For this review, take the finished solid that the model builds, in its own axes (mm). Face numbers are marked on the shaded views. A direction names the side the tool comes from. Give positions to 0.01 mm unless a question says otherwise; leave off trailing zeros. Loops run counter-clockwise (first coordinate to the right, second up) from the corner with the lowest first, then second, coordinate; pieces in that order, holes last. Notation, with made-up numbers: (-7.75, 27.25) - (3.25, 27.25) arc R21 ccw to (3.25, 58.25) - close; hole circle Ø3 at (72.25, 51.25). An arc over 180 degrees is marked (long way). Put each result on its own line as item: value.
from build123d import *

# Parameters (mm, degrees)
EXTRUDE_1_DEPTH     = 1.5
EXTRUDE_3_DEPTH     = 14
SKETCH_4_R          = 1.1
EXTRUDE_4_DEPTH     = 3.2
SKETCH_5_R          = 1.1
EXTRUDE_5_DEPTH     = 3.2
SKETCH_8_R          = 1.1
EXTRUDE_7_DEPTH     = 3.2
SKETCH_9_R          = 0.6
CUT_EXTRUDE_5_DEPTH = 1.5
CUT_EXTRUDE_6_DEPTH = 1.5
CUT_EXTRUDE_7_REACH = 88.953
SKETCH_16_R         = 3.5
FILLET_1_R          = 1


with BuildPart() as part:
    # 草图1 → 凸台-拉伸1 (new body)
    with BuildSketch(Plane.XY):
        with BuildLine():
            Line((-3.146845785, 60.5), (38.953154215, 60.5))
            ThreePointArc((38.953154215, 60.5), (45.458536602, 57.805382387), (48.153154215, 51.3))
            Line((48.153154215, 51.3), (48.153154215, 9.2))
            ThreePointArc((48.153154215, 9.2), (45.458536602, 2.694617613), (38.953154215, 0))
            Line((38.953154215, 0), (-3.146845785, 0))
            ThreePointArc((-3.146845785, 0), (-9.652228172, 2.694617613), (-12.346845785, 9.2))
            Line((-12.346845785, 9.2), (-12.346845785, 51.3))
            ThreePointArc((-12.346845785, 51.3), (-9.652228172, 57.805382387), (-3.146845785, 60.5))
        make_face()
    extrude(amount=EXTRUDE_1_DEPTH)

    # 草图3 → 凸台-拉伸3 (add)
    with BuildSketch(Plane.XY.offset(1.5)):
        with BuildLine():
            Line((38.953154215, 60.5), (-3.146845785, 60.5))
            ThreePointArc((-3.146845785, 60.5), (-9.652228172, 57.805382387), (-12.346845785, 51.3))
            Line((-12.346845785, 51.3), (-12.346845785, 9.2))
            ThreePointArc((-12.346845785, 9.2), (-9.652228172, 2.694617613), (-3.146845785, 0))
            Line((-3.146845785, 0), (38.953154215, 0))
            ThreePointArc((38.953154215, 0), (45.458536602, 2.694617613), (48.153154215, 9.2))
            Line((48.153154215, 9.2), (48.153154215, 51.3))
            ThreePointArc((48.153154215, 51.3), (45.458536602, 57.805382387), (38.953154215, 60.5))
        make_face()
        with BuildLine():
            Line((38.953154215, 59), (-3.146845785, 59))
            ThreePointArc((-3.146845785, 59), (-8.591568001, 56.744722215), (-10.846845785, 51.3))
            Line((-10.846845785, 51.3), (-10.846845785, 9.2))
            ThreePointArc((-10.846845785, 9.2), (-8.591568001, 3.755277785), (-3.146845785, 1.5))
            Line((-3.146845785, 1.5), (38.953154215, 1.5))
            ThreePointArc((38.953154215, 1.5), (44.39787643, 3.755277785), (46.653154215, 9.2))
            Line((46.653154215, 9.2), (46.653154215, 51.3))
            ThreePointArc((46.653154215, 51.3), (44.39787643, 56.744722215), (38.953154215, 59))
        make_face(mode=Mode.SUBTRACT)
    extrude(amount=EXTRUDE_3_DEPTH)

    # 草图4 → 凸台-拉伸4 (add)
    with BuildSketch(Plane.XY.offset(1.5)):
        with BuildLine():
            Line((0, 52), (0, 59))
            Line((0, 59), (-3.146845785, 59))
            ThreePointArc((-3.146845785, 59), (-8.591568001, 56.744722215), (-10.846845785, 51.3))
            Line((-10.846845785, 51.3), (-10.846845785, 49))
            Line((-10.846845785, 49), (-3, 49))
            ThreePointArc((-3, 49), (-0.878679656, 49.878679656), (0, 52))
        make_face()
        with Locations((-4.646845785, 52.8)):
            Circle(SKETCH_4_R, mode=Mode.SUBTRACT)
    extrude(amount=EXTRUDE_4_DEPTH)

    # 草图5 → 凸台-拉伸5 (add)
    with BuildSketch(Plane.XY.offset(1.5)):
        with BuildLine():
            Line((-4.846845785, 10.5), (-10.846845785, 10.5))
            Line((-10.846845785, 10.5), (-10.846845785, 9.2))
            ThreePointArc((-10.846845785, 9.2), (-8.591568001, 3.755277785), (-3.146845785, 1.5))
            Line((-3.146845785, 1.5), (-1.846845785, 1.5))
            Line((-1.846845785, 1.5), (-1.846845785, 7.5))
            ThreePointArc((-1.846845785, 7.5), (-2.725525442, 9.621320344), (-4.846845785, 10.5))
        make_face()
        with Locations((-4.646845785, 8.3)):
            Circle(SKETCH_5_R, mode=Mode.SUBTRACT)
    extrude(amount=EXTRUDE_5_DEPTH)

    # 草图8 → 凸台-拉伸7 (add)
    with BuildSketch(Plane.XY.offset(1.5)):
        with BuildLine():
            Line((37.653154215, 7.5), (37.653154215, 1.5))
            Line((37.653154215, 1.5), (38.953154215, 1.5))
            ThreePointArc((38.953154215, 1.5), (44.39787643, 3.755277785), (46.653154215, 9.2))
            Line((46.653154215, 9.2), (46.653154215, 10.5))
            Line((46.653154215, 10.5), (40.653154215, 10.5))
            ThreePointArc((40.653154215, 10.5), (38.531833871, 9.621320344), (37.653154215, 7.5))
        make_face()
        with Locations((40.453154215, 8.3)):
            Circle(SKETCH_8_R, mode=Mode.SUBTRACT)
    extrude(amount=EXTRUDE_7_DEPTH)

    # 草图9 → 切除-拉伸5 (cut)
    with BuildSketch(Plane.ZY.offset(12.346845785)):
        with Locations(Location((8, 32.8, 0), (0, 0, 270))):
            Circle(SKETCH_9_R)
    extrude(amount=-CUT_EXTRUDE_5_DEPTH, mode=Mode.SUBTRACT)

    # 草图10 → 切除-拉伸6 (cut)
    with BuildSketch(Plane.ZY.offset(12.346845785)):
        with BuildLine():
            Line((9.5, 20.4), (9.5, 14.4))
            ThreePointArc((9.5, 14.4), (7.75, 12.65), (6, 14.4))
            Line((6, 14.4), (6, 20.4))
            ThreePointArc((6, 20.4), (7.75, 22.15), (9.5, 20.4))
        make_face()
    extrude(amount=-CUT_EXTRUDE_6_DEPTH, mode=Mode.SUBTRACT)

    # 草图16 → 切除-拉伸7 (cut, up to next)
    with BuildSketch(Plane(origin=(48.153154215, 0, 0), x_dir=(0, 0, -1), z_dir=(1, 0, 0)), mode=Mode.PRIVATE) as cut_extrude_7_sk1:
        with Locations((-9.65, 27.1)):
            Circle(SKETCH_16_R)
    cut_extrude_7_tool1 = extrude(cut_extrude_7_sk1.sketch, amount=-CUT_EXTRUDE_7_REACH, mode=Mode.PRIVATE) & part.part
    # 草图16 → 切除-拉伸7 (cut, up to next)
    with BuildSketch(Plane(origin=(48.153154215, 0, 0), x_dir=(0, 0, -1), z_dir=(1, 0, 0)), mode=Mode.PRIVATE) as cut_extrude_7_sk2:
        with BuildLine():
            Line((-12, 40.8), (-8, 40.8))
            ThreePointArc((-8, 40.8), (-6.585786438, 40.214213562), (-6, 38.8))
            Line((-6, 38.8), (-6, 35))
            ThreePointArc((-6, 35), (-6.585786438, 33.585786438), (-8, 33))
            Line((-8, 33), (-12, 33))
            ThreePointArc((-12, 33), (-13.414213562, 33.585786438), (-14, 35))
            Line((-14, 35), (-14, 38.8))
            ThreePointArc((-14, 38.8), (-13.414213562, 40.214213562), (-12, 40.8))
        make_face()
    cut_extrude_7_tool2 = extrude(cut_extrude_7_sk2.sketch, amount=-CUT_EXTRUDE_7_REACH, mode=Mode.PRIVATE) & part.part
    add(cut_extrude_7_tool1.solids().sort_by_distance((48.153154, 27.1, 9.65))[0], mode=Mode.SUBTRACT)
    add(cut_extrude_7_tool2.solids().sort_by_distance((48.153154, 36.9, 10))[0], mode=Mode.SUBTRACT)

    # 圆角1
    fillet_1_edges = [part.edges().sort_by_distance(p)[0] for p in [
        (-12.346845785, 30.25, 0),
        (-9.652228172, 57.805382387, 0),
        (17.903154215, 60.5, 0),
        (45.458536602, 57.805382387, 0),
        (48.153154215, 30.25, 0),
        (45.458536602, 2.694617613, 0),
        (17.903154215, 0, 0),
        (-9.652228172, 2.694617613, 0),
    ]]
    fillet(fillet_1_edges, radius=FILLET_1_R)


solid = part.part
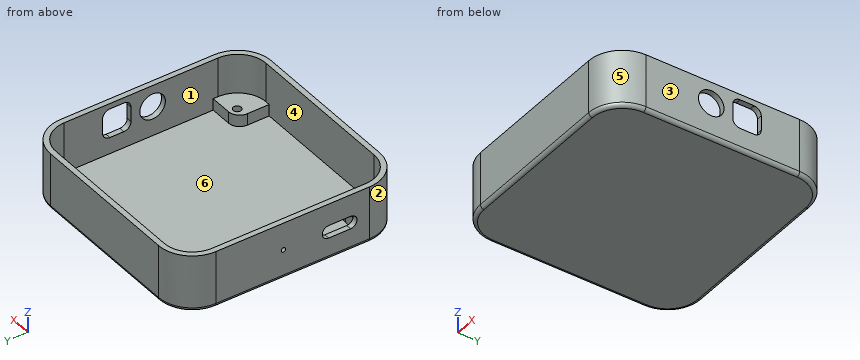
1) Insertion check: pin 1 Ø1.6 at (x, z) = (47.5, 10) entering from -Y; pin 2 Ø6 at (x, y) = (13.5, 45) entering from +Z; pin 3 Ø7 at (y, z) = (33.5, 9) entering from +X; pin 4 Ø3.5 at (y, z) = (4, 3.5) entering from +X. Each pin has a flat end and moves straight along its axis. Give the tip position at first contact, or say it passes through.
Geometry check:
pin 1: stops at y = 4.24
pin 2: stops at z = 1.5
pin 3: stops at x = 48.15
pin 4: stops at x = 47.48
2) For the marked faces 1 and 2, list the 3-axis set-ups (+Z, -Z, +X, -X, +Y, -Y) from which the entire face can be reached by the end or side of a thin tool; tool diameter is ignored.
Geometry check:
face 1: +Z
face 2: +Z, -Z, -X, -Y
3) Wall thickness on line 1 (Y direction, x = 25.5, z = 5.75); line 2 (X direction, y = 46.5, z = 4.75); line 3 (Z direction, x = 17.5, y = 28.5): over which ranges is each line inside the solid? List them lowest first.
Geometry check:
line 1: y = 0 to 1.5, 59 to 60.5
line 2: x = -12.35 to -10.85, 46.65 to 48.15
line 3: z = 0 to 1.5
4) Take a section at A-A on z = 2.75. State the section outline as (x, y) points, and give its area (3 significant figures).
Geometry check:
outline: (-12.35, 9.2) arc R9.2 ccw to (-3.15, 0) - (38.95, 0) arc R9.2 ccw to (48.15, 9.2) - (48.15, 51.3) arc R9.2 ccw to (38.95, 60.5) - (-3.15, 60.5) arc R9.2 ccw to (-12.35, 51.3) - close; hole (-10.85, 10.5) - (-4.85, 10.5) arc R3 cw to (-1.85, 7.5) - (-1.85, 1.5) - (37.65, 1.5) - (37.65, 7.5) arc R3 cw to (40.65, 10.5) - (46.65, 10.5) - (46.65, 51.3) arc R7.7 ccw to (38.95, 59) - (0, 59) - (0, 52) arc R3 cw to (-3, 49) - (-10.85, 49) - close; hole circle Ø2.2 at (-4.65, 8.3); hole circle Ø2.2 at (-4.65, 52.8); hole circle Ø2.2 at (40.45, 8.3)
area: 547 mm²
5) Draft analysis for pull direction Y (two halves, no side actions). For the marked faces 3, 4, 5 and 6, state which applies: pulls with the +Y half, pulls with the -Y half, needs draft (parallel to the pull), parting line crosses it, or undercut.
Geometry check:
face 3: needs draft
face 4: undercut
face 5: pulls with the -Y half
face 6: undercut
6) Take a section at B-B on y = 45. State the section outline as (x, z) points.
Geometry check:
outline: (-12.35, 1) arc R1 ccw to (-11.35, 0) - (47.15, 0) arc R1 ccw to (48.15, 1) - (48.15, 15.5) - (46.65, 15.5) - (46.65, 1.5) - (-10.85, 1.5) - (-10.85, 15.5) - (-12.35, 15.5) - close
7) Take a section at C-C on x = 33. State the section outline as (y, z) points.
Geometry check:
outline: (0, 1) arc R1 ccw to (1, 0) - (59.5, 0) arc R1 ccw to (60.5, 1) - (60.5, 15.5) - (59, 15.5) - (59, 1.5) - (1.5, 1.5) - (1.5, 15.5) - (0, 15.5) - close
